Print and shaded views of the part. All mm, measured from the part's lowest x, y and z. A direction names the side the tool comes from. Give positions to 0.01 mm unless a question says otherwise; leave off trailing zeros. Loops run counter-clockwise (first coordinate to the right, second up) from the corner with the lowest first, then second, coordinate; pieces in that order, holes last. Notation, with made-up numbers: M -22.5,-14.5 L -11.5,-14.5 A31 ccw -11.5,11.5 Z; hole C 11.5,29 d2. An arc over 180 degrees is marked long. Answer as CSV lines item,"result".
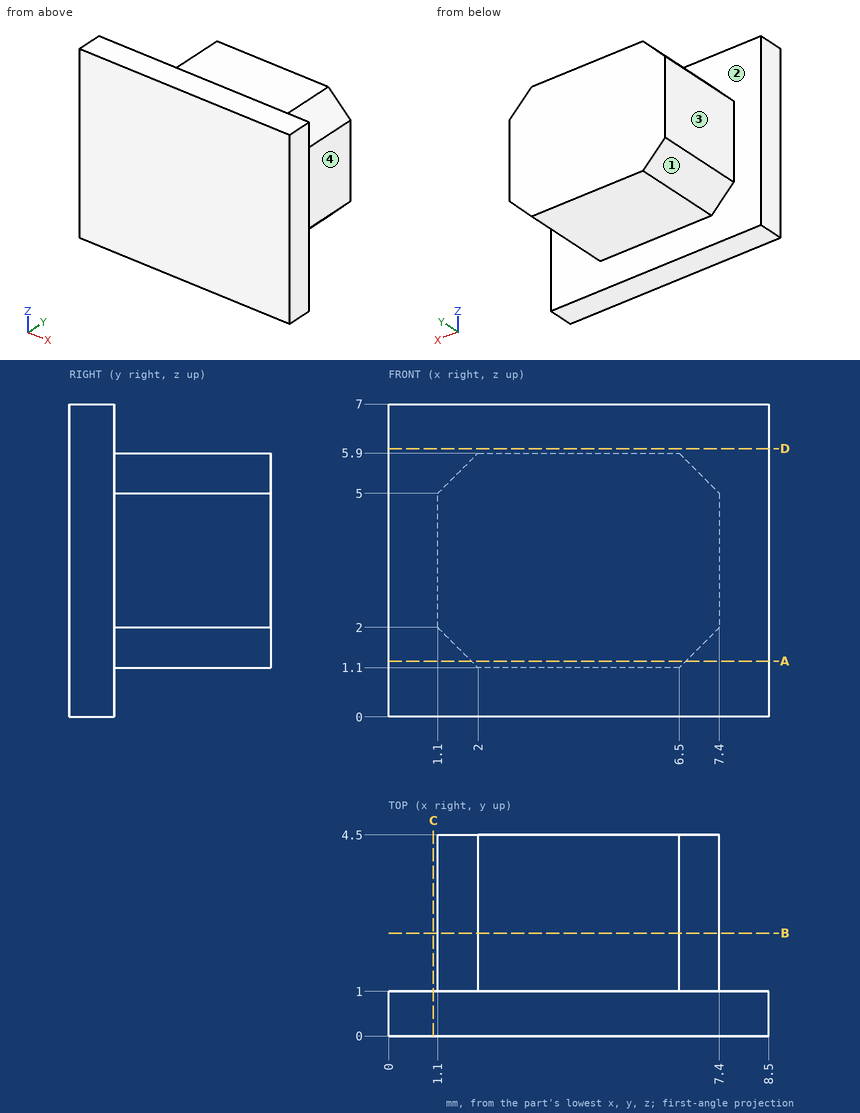
Q1. Cut at C-C (x = 1). Write the cut outline in (y, z).
Solution:
outline,"M 0,0 L 1,0 L 1,7 L 0,7 Z"
Q2. Pin check, flat tips, straight feed: P1, Ø1, axis at x = 7.5, z = 5, coming from the +Y side; P2, Ø2.5, axis at y = 3, z = 4, coming from the +X side; P3, Ø1.8, axis at x = 3, y = 2, coming from the +Z side; P4, Ø2.5, axis at y = 2.5, z = 3.5, coming from the -X side. Stop position of each tip, or through.
Solution:
P1,"stops at y = 4.5"
P2,"stops at x = 7.4"
P3,"stops at z = 5.9"
P4,"stops at x = 1.1"
Q3. Wall check: line 1 (Y direction, x = 7.5, z = 6); line 2 (Z direction, x = 3.25, y = 3.4); line 3 (X direction, y = 3.3, z = 2.5). Give the ranges that are in metal, low to high. Write a range as [from, to].
Solution:
line 1,"y = [0, 1]"
line 2,"z = [1.1, 5.9]"
line 3,"x = [1.1, 7.4]"
Q4. Cut at A-A (z = 1.25). Write the cut outline in (x, y), and give its area (3 significant figures).
Solution:
outline,"M 0,0 L 8.5,0 L 8.5,1 L 6.65,1 L 6.65,4.5 L 1.85,4.5 L 1.85,1 L 0,1 Z"
area,"25.3 mm²"
Q5. Which spindle directions (+Z, -Z, +X, -X, +Y, -Y) get a long thin tool onto all of the face, cutting with end or side? Do the marked faces 1, 2, 3 and 4. Say none if no direction does.
Solution:
face 1,"-Z, -X, +Y"
face 2,"+Y"
face 3,"+Z, -Z, -X, +Y"
face 4,"+Z, -Z, +X, +Y"
Q6. Cut at B-B (y = 2.3). Write the cut outline in (x, z), and give its area (3 significant figures).
Solution:
outline,"M 1.1,2 L 2,1.1 L 6.5,1.1 L 7.4,2 L 7.4,5 L 6.5,5.9 L 2,5.9 L 1.1,5 Z"
area,"28.6 mm²"
Q7. Cut at D-D (z = 6). Write the cut outline in (x, y), and give its area (3 significant figures).
Solution:
outline,"M 0,0 L 8.5,0 L 8.5,1 L 0,1 Z"
area,"8.50 mm²"
